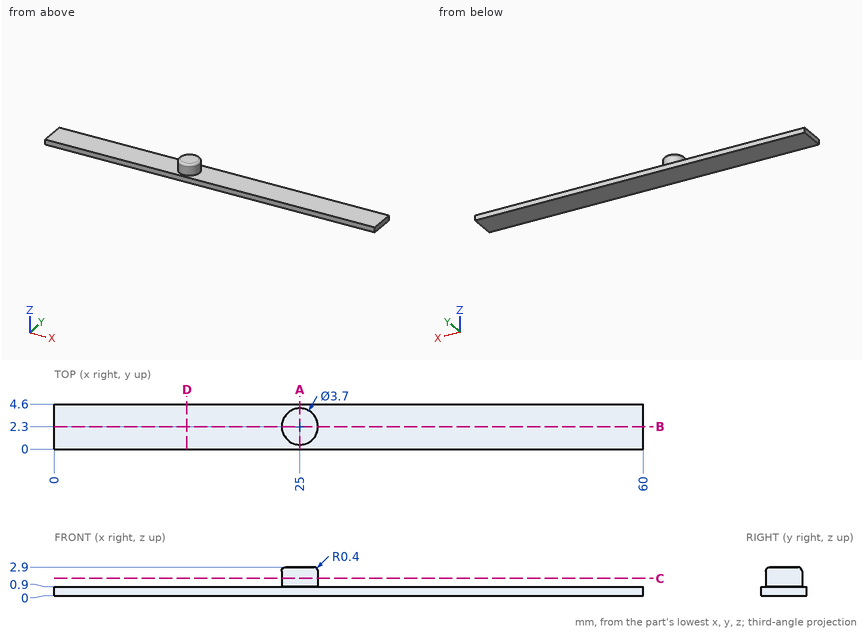
For this review, use the dimensioned drawing (mm, ordinates from the lowest corner) and the shaded views. Round coordinates to 2 decimals unless told otherwise and drop trailing zeros. Order: outer loops, then holes, each group sorted by start corner. A loop starts at its lowest first (then second) coordinate and runs counter-clockwise, first axis right, second up. Notation, with made-up numbers: M 79.25,-13.5 L 90.25,-13.5 A22 ccw 90.25,16.5 Z; hole C 77.5,56 d10. An arc over 180 degrees is marked long. Use a Markdown table: item, result.
1) Consider section D-D (x = 13.5). Write out the cut boundary in (y, z), then the cut area to 3 significant figures.
Report:
| item | result |
|---|---|
| outline | M 0,0 L 4.6,0 L 4.6,0.9 L 0,0.9 Z |
| area | 4.14 mm^2 |
2) Wall thickness on line 1 along Z through (x, y) = (17.5, 4.35); line 2 along X through (y, z) = (1.2, 1.3): over which ranges is each line inside the solid? List them lowest first. Write a range as [from, to].
Report:
| item | result |
|---|---|
| line 1 | [0, 0.9] |
| line 2 | [23.51, 26.49] |
3) Consider section C-C (z = 1.75). Write out the cut boundary in (x, y), then the cut area to 3 significant figures.
Report:
| item | result |
|---|---|
| outline | C 25,2.3 d3.7 |
| area | 10.8 mm^2 |
4) Consider section A-A (x = 25). Write out the cut boundary in (y, z).
Report:
| item | result |
|---|---|
| outline | M 0,0 L 4.6,0 L 4.6,0.9 L 4.15,0.9 L 4.15,2.5 A0.4 ccw 3.75,2.9 L 0.85,2.9 A0.4 ccw 0.45,2.5 L 0.45,0.9 L 0,0.9 Z |
5) Insertion check: pin 1 (1 mm diameter, centred on x = 34.5, y = 0.5, fed in from +Z); pin 2 (1.5 mm diameter, centred on y = 4, z = 2.5, fed in from +X). Each pin has a flat end and moves straight along its axis. Give the tip position at first contact, or say it passes through.
Report:
| item | result |
|---|---|
| pin 1 | z = 0.9 |
| pin 2 | x = 26.59 |
6) Consider section B-B (y = 2.3). Write out the cut boundary in (x, z), then the cut area to 3 significant figures.
Report:
| item | result |
|---|---|
| outline | M 0,0 L 60,0 L 60,0.9 L 26.85,0.9 L 26.85,2.5 A0.4 ccw 26.45,2.9 L 23.55,2.9 A0.4 ccw 23.15,2.5 L 23.15,0.9 L 0,0.9 Z |
| area | 61.3 mm^2 |
